```python
from build123d import *

# Parameters (mm, degrees)
SKETCH_W            = 30
SKETCH_H            = 11.6
PAD_DEPTH           = 8
SKETCH001_R         = 2.6
POCKET_DEPTH        = 0.001
POCKET_DEPTH_BACK   = 8.001
LINEARPATTERN_COUNT = 4
LINEARPATTERN_PITCH = 6.666667
PARTDESIGN_FILLET_R = 0.5


with BuildPart() as part:
    # Sketch → Pad (new body)
    with BuildSketch(Plane.XY):
        Rectangle(SKETCH_W, SKETCH_H)
    extrude(amount=PAD_DEPTH)

    # Sketch001 → Pocket (cut, two sides)
    with BuildSketch(Plane.XY) as pocket_sk:
        with Locations((-10, 3.46)):
            Circle(SKETCH001_R)
        with Locations((-10, -3.46)):
            Circle(SKETCH001_R)
    pocket = extrude(amount=-POCKET_DEPTH, mode=Mode.SUBTRACT) + extrude(pocket_sk.sketch, amount=POCKET_DEPTH_BACK, mode=Mode.SUBTRACT)

    # LinearPattern: Pocket ×4
    with Locations(*[(i * LINEARPATTERN_PITCH, 0, 0) for i in range(1, LINEARPATTERN_COUNT)]):
        add(pocket, mode=Mode.SUBTRACT)

    # PartDesign__Fillet
    partdesign_fillet_edges = [part.edges().sort_by_distance(p)[0] for p in [
        (-15, -5.8, 4),
        (-15, 5.8, 4),
        (-11.133314, -5.8, 4),
        (-11.133314, 5.8, 4),
        (-7.4, -3.46, 4),
        (-7.4, 3.46, 4),
        (-8.866686, 5.8, 4),
        (-4.466647, 5.8, 4),
        (-0.733333, 3.46, 4),
        (-2.20002, 5.8, 4),
        (2.20002, 5.8, 4),
        (5.933333, 3.46, 4),
        (4.466647, 5.8, 4),
        (8.866686, 5.8, 4),
        (12.6, 3.46, 4),
        (11.133314, 5.8, 4),
        (15, 5.8, 4),
        (15, -5.8, 4),
        (11.133314, -5.8, 4),
        (12.6, -3.46, 4),
        (8.866686, -5.8, 4),
        (4.466647, -5.8, 4),
        (5.933333, -3.46, 4),
        (2.20002, -5.8, 4),
        (-2.20002, -5.8, 4),
        (-0.733333, -3.46, 4),
        (-4.466647, -5.8, 4),
        (-8.866686, -5.8, 4),
    ]]
    fillet(partdesign_fillet_edges, radius=PARTDESIGN_FILLET_R)


solid = part.part
```
Input: part model. Units: mm. Frame: model coordinates. Give positions to 0.01 mm unless a question says otherwise; leave off trailing zeros. Order: outer loops, then holes, each group sorted by start corner. A loop starts at its lowest first (then second) coordinate and runs counter-clockwise, first axis right, second up. Notation, with made-up numbers: (7, 24.25) -> (14, 24.25) arc R13 cw to (14, 45.25) -> close; hole circle Ø8 at (-31, -38). An arc over 180 degrees is marked (long way). Write each question's results on one line, items separated by ' | '. Start each with the question number.
Item 1: Mould query, pull axis X, two halves, no side actions, for faces 1 (the cylindrical face through (-3.41, 0.86, 4.06)), 2 (the flat face through (15, 0, 4)), 3 (the flat face through (0, 5.8, 4)), 4 (the cylindrical face through (-9.92, -0.86, 3.94)). Classes: pulls with the +X half, pulls with the -X half, needs draft (parallel to the pull), parting line crosses it, or undercut.
Item 2: Cut plane C-C on y = 4.5. Return the cut outline in (x, z), then the cut area to 3 significant figures.
Item 3: Line query: line 1 (X direction, y = 3.46, z = 5.5); line 2 (X direction, y = -2.75, z = 6.5); line 3 (Y direction, x = -10, z = 2.75). Output: solid intervals per line, ascending.
Item 4: Cut plane A-A on y = -3.46. Return the cut outline in (x, z), then the cut area to 3 significant figures.
Item 5: Cut plane D-D on x = 9.5. Return the cut outline in (y, z), then the cut area to 3 significant figures.
Item 6: Contact query for a flat-ended pin moving along its axis: P1, Ø4, axis at x = -3.33, y = 3.46, coming from the +Z side. Output: stop coordinate, or through.
Item 7: Cut plane B-B on x = -10. Return the cut outline in (y, z), then the cut area to 3 significant figures.
Established:
1) face 1: undercut | face 2: pulls with the +X half | face 3: needs draft | face 4: undercut
2) outline: (-15, 0) -> (-12.38, 0) -> (-12.38, 8) -> (-15, 8) -> close; (-7.62, 0) -> (-5.72, 0) -> (-5.72, 8) -> (-7.62, 8) -> close; (-0.95, 0) -> (0.95, 0) -> (0.95, 8) -> (-0.95, 8) -> close; (5.72, 0) -> (7.62, 0) -> (7.62, 8) -> (5.72, 8) -> close; (12.38, 0) -> (15, 0) -> (15, 8) -> (12.38, 8) -> close | area: 87.5 mm^2
3) line 1: -15 to -12.6, -7.4 to -5.93, -0.73 to 0.73, 5.93 to 7.4, 12.6 to 15 | line 2: -15 to -12.5, -7.5 to -5.83, -0.83 to 0.83, 5.83 to 7.5, 12.5 to 15 | line 3: -0.86 to 0.86
4) outline: (-15, 0) -> (-12.6, 0) -> (-12.6, 8) -> (-15, 8) -> close; (-7.4, 0) -> (-5.93, 0) -> (-5.93, 8) -> (-7.4, 8) -> close; (-0.73, 0) -> (0.73, 0) -> (0.73, 8) -> (-0.73, 8) -> close; (5.93, 0) -> (7.4, 0) -> (7.4, 8) -> (5.93, 8) -> close; (12.6, 0) -> (15, 0) -> (15, 8) -> (12.6, 8) -> close | area: 73.6 mm^2
5) outline: (-0.91, 0) -> (0.91, 0) -> (0.91, 8) -> (-0.91, 8) -> close | area: 14.5 mm^2
6) P1: through
7) outline: (-0.86, 0) -> (0.86, 0) -> (0.86, 8) -> (-0.86, 8) -> close | area: 13.8 mm^2
